Geometry check sheet. Reference: the model listing, model coordinates, mm. Face numbers are marked on the shaded views. A direction names the side the tool comes from. Coordinates: 2 decimals unless noted, no trailing zeros. Order: outer loops, then holes, each group sorted by start corner. A loop starts at its lowest first (then second) coordinate and runs counter-clockwise, first axis right, second up. Notation, with made-up numbers: (52, 17) - (105, 17) arc R16 cw to (105, 23) - close; hole circle Ø8 at (75.25, 9). An arc over 180 degrees is marked (long way). Use CSV: the item, a comma, the result in double quotes. Start each with the question number.
1) Draft check along X on the marked faces 1, 2 and 3. Enter one of: released by +X, released by -X, zero draft, split by the parting line, or undercut.
2) Depth check by flat-ended pin: P1, Ø4.5, axis at y = 47, z = 10, coming from the -X side; P2, Ø5.5, axis at x = 1, y = 8, coming from the +Z side; P3, Ø7.5, axis at x = -30, z = 7, coming from the -Y side; P4, Ø4.5, axis at x = 13, y = 5.5, coming from the -Z side. Enter the tip coordinate at first touch or a pass-through.
3) Sectioned sample at D-D, the plane y = 85.5. Record the cut outline in (x, z).
4) Thickness scan on probe 1 along X at (y, z) = (4, 11.5); probe 2 along Y at (x, z) = (-13, 7.5); probe 3 along Z at (x, y) = (25, 90). Record the ranges inside material, lowest first. Write a range as [from, to].
5) Sectioned sample at C-C, the plane y = 9.5. Record the cut outline in (x, z), and give its area (3 significant figures).
6) Sectioned sample at A-A, the plane x = 0. Record the cut outline in (y, z).
7) Tool access check on the marked faces 4, 5 and 6. Record the directions out of +Z, -Z, +X, -X, +Y, -Y that give a thin tool (end or side, any length) a straight path to the whole face; none if there is none.
8) Sectioned sample at B-B, the plane y = 69. Record the cut outline in (x, z).
from build123d import *

# Parameters (mm, degrees)
ESTRUSIONE_ESTRUSIONE1_DEPTH                         = 15
FORO_5_0_5_1_D                                       = 5
FORO_5_0_5_1_DEPTH                                   = 16
FORO_5_0_5_1_TIP                                     = 1.502151548
FORO_FILETTATO_M6_1_D                                = 5
FORO_FILETTATO_M6_1_DEPTH                            = 20
FORO_FILETTATO_M6_1_TIP                              = 1.502151548
SCHIZZO7_R                                           = 6
TAGLIO_ESTRUSIONE1_DEPTH                             = 16.5
FORO_5_0_5_2_D                                       = 5
FORO_LAMATO_PER_VITE_M6_A_TESTA_CILINDRI_D           = 6.6
FORO_LAMATO_PER_VITE_M6_A_TESTA_CILINDRI_CBORE_D     = 11
FORO_LAMATO_PER_VITE_M6_A_TESTA_CILINDRI_CBORE_DEPTH = 6.4
SMUSSO1_SIZE                                         = 1
SMUSSO2_SIZE                                         = 0.5


with BuildPart() as part:
    # Schizzo1 → Estrusione-Estrusione1 (new body)
    with BuildSketch(Plane.XY):
        Polygon((19, 0), (-19, 0), (-19, 15), (-40, 15), (-40, 25), (-32.432495061, 97), (-12, 97), (-12, 60), (-8, 60), (-8, 36), (8, 36), (8, 60), (12, 60), (12, 97), (32.432495061, 97), (40, 25), (40, 15), (19, 15), align=None)
    extrude(amount=ESTRUSIONE_ESTRUSIONE1_DEPTH)

    # Foro Ø5.0 (5)-1
    with Locations(Plane(origin=(0, 97, 0), x_dir=(1, 0, 0), z_dir=(0, 1, 0))):
        with Locations((-16, -7.5), (16, -7.5)):
            Hole(FORO_5_0_5_1_D / 2, depth=FORO_5_0_5_1_DEPTH)
            with Locations((0, 0, -(FORO_5_0_5_1_DEPTH + FORO_5_0_5_1_TIP / 2))):  # 118° drill point
                Cone(0, FORO_5_0_5_1_D / 2, FORO_5_0_5_1_TIP, mode=Mode.SUBTRACT)

    # Foro filettato M6-1
    with Locations(Plane(origin=(0, 97, 0), x_dir=(1, 0, 0), z_dir=(0, 1, 0))):
        with Locations((-25, -7.5), (25, -7.5)):
            Hole(FORO_FILETTATO_M6_1_D / 2, depth=FORO_FILETTATO_M6_1_DEPTH)
            with Locations((0, 0, -(FORO_FILETTATO_M6_1_DEPTH + FORO_FILETTATO_M6_1_TIP / 2))):  # 118° drill point
                Cone(0, FORO_FILETTATO_M6_1_D / 2, FORO_FILETTATO_M6_1_TIP, mode=Mode.SUBTRACT)

    # Schizzo7 → Taglio-Estrusione1 (cut)
    with BuildSketch(Plane(origin=(0, 36, 0), x_dir=(1, 0, 0), z_dir=(0, 1, 0))):
        with Locations(Location((0, -7.5, 0), (0, 0, 270))):
            Circle(SCHIZZO7_R)
    extrude(amount=-TAGLIO_ESTRUSIONE1_DEPTH, mode=Mode.SUBTRACT)

    # Foro Ø5.0 (5)-2 (through all)
    with Locations(Plane(origin=(0, 0, 0), x_dir=(-1, 0, 0), z_dir=(0, 0, -1))):
        with Locations((-13, 5.5), (13, 9.5)):
            Hole(FORO_5_0_5_2_D / 2)

    # Foro lamato per Vite M6 a testa cilindrica-1 (through all)
    with Locations(Plane.XY.offset(15)):
        with Locations((0, 7.5)):
            CounterBoreHole(FORO_LAMATO_PER_VITE_M6_A_TESTA_CILINDRI_D / 2, FORO_LAMATO_PER_VITE_M6_A_TESTA_CILINDRI_CBORE_D / 2, FORO_LAMATO_PER_VITE_M6_A_TESTA_CILINDRI_CBORE_DEPTH)

    # Smusso1
    smusso1_edges = [part.edges().sort_by_distance(p)[0] for p in [
        (-19, 7.5, 15),
        (19, 7.5, 15),
        (19, 7.5, 0),
        (-19, 7.5, 0),
    ]]
    chamfer(smusso1_edges, length=SMUSSO1_SIZE)

    # Smusso2
    smusso2_edges = [part.edges().sort_by_distance(p)[0] for p in [
        (-12, 78.5, 0),
        (12, 78.5, 0),
    ]]
    chamfer(smusso2_edges, length=SMUSSO2_SIZE)


solid = part.part
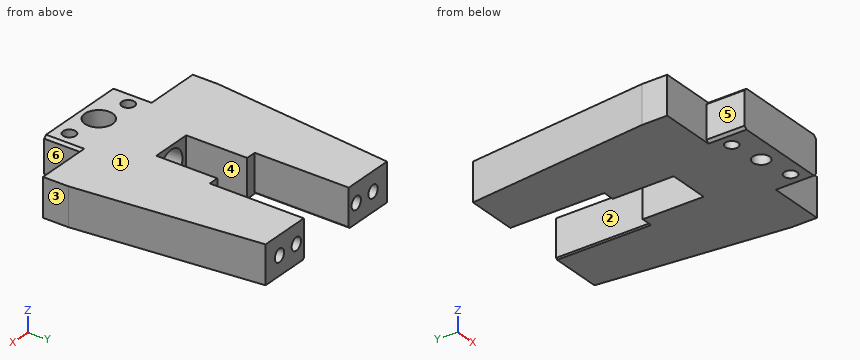
Evaluation:
1,face 1,"zero draft"
1,face 2,"undercut"
1,face 3,"released by +X"
2,P1,"x = -37.92"
2,P2,"z = 8.6"
2,P3,"y = 15"
2,P4,"through"
3,outline,"(-33.64, 0) - (-12.5, 0) - (-12, 0.5) - (-12, 15) - (-33.64, 15) - close; (12, 0.5) - (12.5, 0) - (33.64, 0) - (33.64, 15) - (12, 15) - close; hole circle Ø5 at (-25, 7.5); hole circle Ø5 at (-16, 7.5); hole circle Ø5 at (16, 7.5); hole circle Ø5 at (25, 7.5)"
4,probe 1,"[-19, -4.24], [4.24, 11], [15, 19]"
4,probe 2,"[0, 7], [12, 97]"
4,probe 3,"[0, 5], [10, 15]"
5,outline,"(-19, 1) - (-18, 0) - (-15.5, 0) - (-15.5, 15) - (-18, 15) - (-19, 14) - close; (-10.5, 0) - (-2.62, 0) - (-2.62, 8.6) - (-5.12, 8.6) - (-5.12, 15) - (-10.5, 15) - close; (2.62, 0) - (18, 0) - (19, 1) - (19, 14) - (18, 15) - (5.12, 15) - (5.12, 8.6) - (2.62, 8.6) - close"
5,area,"382 mm²"
6,outline,"(0, 0) - (4.2, 0) - (4.2, 8.6) - (2, 8.6) - (2, 15) - (0, 15) - close; (10.8, 0) - (36, 0) - (36, 1.5) - (19.5, 1.5) - (19.5, 13.5) - (36, 13.5) - (36, 15) - (13, 15) - (13, 8.6) - (10.8, 8.6) - close"
7,face 4,"+Z, -Z, +Y"
7,face 5,"+Z, -Z, -X, -Y"
7,face 6,"+Z, -Z, +X, -Y"
8,outline,"(-35.38, 0) - (-12.5, 0) - (-12, 0.5) - (-12, 15) - (-35.38, 15) - close; (12, 0.5) - (12.5, 0) - (35.38, 0) - (35.38, 15) - (12, 15) - close"
